```python
from build123d import *

# Parameters (mm, degrees)
ESTRUSIONE_ESTRUSIONE1_DEPTH = 50
SCHIZZO2_W                   = 16
SCHIZZO2_H                   = 25
TAGLIO_ESTRUSIONE1_DEPTH     = 6
SCHIZZO3_R                   = 2.25
TAGLIO_ESTRUSIONE2_DEPTH     = 10
SMUSSO1_SIZE                 = 2


with BuildPart() as part:
    # Schizzo1 → Estrusione-Estrusione1 (new body)
    with BuildSketch(Plane.XY):
        Polygon((5, 0), (-5, 0), (-5, -17), (-11, -17), (-11, 8), (11, 8), (11, -17), (5, -17), align=None)
    extrude(amount=ESTRUSIONE_ESTRUSIONE1_DEPTH)

    # Schizzo2 → Taglio-Estrusione1 (cut)
    with BuildSketch(Plane(origin=(11, 0, 0), x_dir=(0, 0, -1), z_dir=(1, 0, 0))):
        with Locations((-25, -4.5)):
            Rectangle(SCHIZZO2_W, SCHIZZO2_H)
    extrude(amount=-TAGLIO_ESTRUSIONE1_DEPTH, mode=Mode.SUBTRACT)

    # Schizzo3 → Taglio-Estrusione2 (cut)
    with BuildSketch(Plane(origin=(-5, 0, 0), x_dir=(0, 0, -1), z_dir=(1, 0, 0))):
        with Locations(Location((-25, -5.5, 0), (0, 0, 90))):
            Circle(SCHIZZO3_R)
    extrude(amount=-TAGLIO_ESTRUSIONE2_DEPTH, mode=Mode.SUBTRACT)

    # Smusso1
    smusso1_edges = [part.edges().sort_by_distance(p)[0] for p in [
        (11, -4.5, 0),
        (11, -4.5, 50),
        (-11, -17, 25),
        (11, -17, 41.5),
        (-11, -4.5, 50),
        (11, -17, 8.5),
        (-11, -4.5, 0),
    ]]
    chamfer(smusso1_edges, length=SMUSSO1_SIZE)


solid = part.part
```
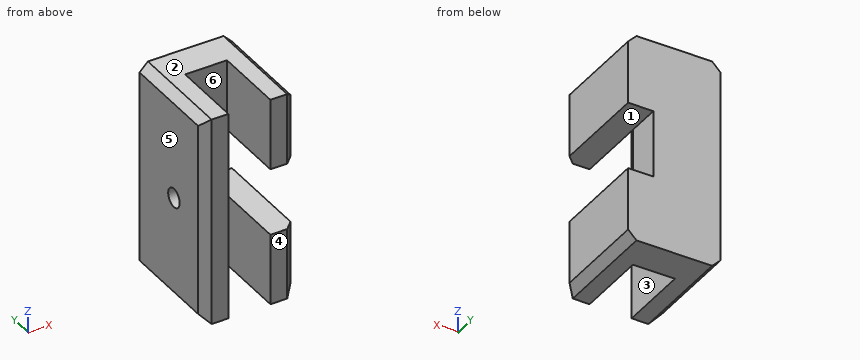
For this review, take the finished solid that the model builds, in its own axes (mm). Face numbers are marked on the shaded views. A direction names the side the tool comes from. Coordinates: 2 decimals unless noted, no trailing zeros. Write each loop counter-clockwise with the first axis right and the second up, starting at its lowest first coordinate (ties: lowest second). Pieces come first, ordered by that corner, then holes. Notation, with made-up numbers: (-16, 43.25) - (41, 43.25) arc R19 ccw to (41, 52.25) - close; hole circle Ø11 at (-27, 48.25). An arc over 180 degrees is marked (long way). Answer in a Markdown table with one row per item. Add a question column.
Q1. We need section D-D, the plane y = -5.5. State the section outline as (x, z) points.
Q2. Tool access review of the marked faces 1, 2 and 3: name each direction out of +Z, -Z, +X, -X, +Y, -Y from which nothing blocks a thin tool from reaching the whole face with its end or side.
Q3. We need section C-C, the plane z = 25. State the section outline as (x, y) points, and give its area (3 significant figures).
Q4. For probe 1 along X at (y, z) = (-4, 42); probe 2 along Z at (x, y) = (-7.95, -5.5); probe 3 along X at (y, z) = (-2.5, 22), list the stretches that pass through material, from the lowest coordinate up.
Q5. We need section B-B, the plane x = 8.25. State the section outline as (y, z) points.
Q6. We need section A-A, the plane y = -11.25. State the section outline as (x, z) points, and give its area (3 significant figures).
Q7. Draft analysis for pull direction X (two halves, no side actions). For the marked faces 4, 5 and 6, state which applies: +X half, -X half, draft (parallel to the pull), parting line (faces both ways), or undercut.
Q8. For P1, Ø4, axis at y = 3, z = 26, coming from the +X side, flat-tipped, find the tip position at first contact; note if it passes through.
Answer list:
| question | item | result |
|---|---|---|
| 1 | outline | (-11, 2) - (-9, 0) - (-5, 0) - (-5, 22.75) - (-11, 22.75) - close; (-11, 27.25) - (-5, 27.25) - (-5, 50) - (-9, 50) - (-11, 48) - close; (5, 0) - (9, 0) - (11, 2) - (11, 17) - (5, 17) - close; (5, 33) - (11, 33) - (11, 48) - (9, 50) - (5, 50) - close |
| 2 | face 1 | +X, +Y, -Y |
| 2 | face 2 | +Z, +X, -X, +Y, -Y |
| 2 | face 3 | +Z, -Z, -Y |
| 3 | outline | (-11, -15) - (-9, -17) - (-5, -17) - (-5, -7.75) - (-11, -7.75) - close; (-11, -3.25) - (-5, -3.25) - (-5, 0) - (5, 0) - (5, 8) - (-11, 8) - close |
| 3 | area | 201 mm2 |
| 4 | probe 1 | x = -11 to -5, 5 to 11 |
| 4 | probe 2 | z = 0 to 22.75, 27.25 to 50 |
| 4 | probe 3 | x = -11 to -5 |
| 5 | outline | (-17, 0) - (8, 0) - (8, 17) - (-17, 17) - close; (-17, 33) - (8, 33) - (8, 50) - (-17, 50) - close |
| 6 | outline | (-11, 2) - (-9, 0) - (-5, 0) - (-5, 50) - (-9, 50) - (-11, 48) - close; (5, 0) - (9, 0) - (11, 2) - (11, 17) - (5, 17) - close; (5, 33) - (11, 33) - (11, 48) - (9, 50) - (5, 50) - close |
| 6 | area | 496 mm2 |
| 7 | face 4 | draft |
| 7 | face 5 | -X half |
| 7 | face 6 | undercut |
| 8 | P1 | stops at x = 5 |
